Source: CAD feature listing. Evaluate the final solid. Frame: model axes, mm. A direction names the side the tool comes from. Round coordinates to 2 decimals unless told otherwise and drop trailing zeros. Order: outer loops, then holes, each group sorted by start corner. A loop starts at its lowest first (then second) coordinate and runs counter-clockwise, first axis right, second up. Notation, with made-up numbers: (19.5, -13.5) - (71.5, -13.5) arc R32 ccw to (71.5, 16.5) - close; hole circle Ø6 at (42.25, 67.25). An arc over 180 degrees is marked (long way). Put each result on its own line as item: value. Start each with the question number.
1) Access query for faces 5 (the face through (0, 0, -4)), 6 (the face through (-20, -46, 1)). Directions: +Z, -Z, +X, -X, +Y, -Y. A direction counts if a zero-diameter tool reaches every point of the face in a straight line with its end or side. Return the directions, or none.
2) Section B-B on z = -2. Output: boundary loops of the cut face in (x, y).
3) Mould query, pull axis Y, two halves, no side actions, for faces 1 (the face through (0, -72, -14)), 2 (the face through (0, 20, 3)), 3 (the face through (0, -75, -3)), 4 (the face through (1.08, -4.88, -1.97)). Classes: +Y half, -Y half, draft (parallel to the pull), parting line (faces both ways), or undercut.
4) Section A-A on z = -7. Output: boundary loops of the cut face in (x, y), then the cut area to 3 significant figures.
5) Line query: probe 1 along X at (y, z) = (-71.4, -7); probe 2 along Z at (x, y) = (10, -72.2); probe 3 along Z at (x, y) = (-10, -2). Output: solid intervals per line, ascending. Write a range as [from, to].
6) Section C-C on x = -10. Output: boundary loops of the cut face in (y, z).
7) Contact query for flat-ended pins moving along their axis: P1, Ø2.5, axis at x = 10, z = -7, coming from the -Y side; P2, Ø4, axis at x = -10, z = -7, coming from the +Y side; P3, Ø11, axis at x = -0.5, y = 0, coming from the -Z side; P4, Ø20, axis at x = -5, y = -34.5, coming from the -Z side. Output: stop coordinate, or through.
8) Section D-D on x = 0. Output: boundary loops of the cut face in (y, z), then the cut area to 3 significant figures.
```python
from build123d import *

# Parameters (mm, degrees)
BOSS_EXTRUDE1_DEPTH = 7
SKETCH2_R           = 5
BOSS_EXTRUDE2_DEPTH = 4
SKETCH3_W           = 40
SKETCH3_H           = 5
BOSS_EXTRUDE3_DEPTH = 14
SKETCH5_R           = 1.5
CUT_EXTRUDE1_DEPTH  = 6


with BuildPart() as part:
    # Sketch1 → Boss-Extrude1 (new body)
    with BuildSketch(Plane.XY):
        with BuildLine():
            Line((20, 0), (20, -75))
            Line((20, -75), (-20, -75))
            Line((-20, -75), (-20, 0))
            ThreePointArc((-20, 0), (0, 20), (20, 0))
        make_face()
    extrude(amount=BOSS_EXTRUDE1_DEPTH)

    # Sketch2 → Boss-Extrude2 (add)
    with BuildSketch(Plane(origin=(0, 0, 0), x_dir=(-1, 0, 0), z_dir=(0, 0, -1))):
        Circle(SKETCH2_R)
    extrude(amount=BOSS_EXTRUDE2_DEPTH)

    # Sketch3 → Boss-Extrude3 (add)
    with BuildSketch(Plane(origin=(0, 0, 0), x_dir=(-1, 0, 0), z_dir=(0, 0, -1))):
        with Locations((0, -72.5)):
            Rectangle(SKETCH3_W, SKETCH3_H)
    extrude(amount=BOSS_EXTRUDE3_DEPTH)

    # Sketch5 → Cut-Extrude1 (cut, through all)
    with BuildSketch(Plane(origin=(0, -70, 0), x_dir=(1, 0, 0), z_dir=(0, 1, 0))):
        with Locations((10, 7)):
            Circle(SKETCH5_R)
        with Locations((-10, 7)):
            Circle(SKETCH5_R)
    extrude(amount=-CUT_EXTRUDE1_DEPTH, mode=Mode.SUBTRACT)


solid = part.part
```
Answer sheet:
1. face 5: -Z, +X, -X, +Y
1. face 6: +Z, -Z, -X, +Y, -Y
2. outline: (-20, -75) - (20, -75) - (20, -70) - (-20, -70) - close; circle Ø10 at (0, 0)
3. face 1: draft
3. face 2: +Y half
3. face 3: -Y half
3. face 4: undercut
4. outline: (-20, -75) - (-11.5, -75) - (-11.5, -70) - (-20, -70) - close; (-8.5, -75) - (8.5, -75) - (8.5, -70) - (-8.5, -70) - close; (11.5, -75) - (20, -75) - (20, -70) - (11.5, -70) - close
4. area: 170 mm^2
5. probe 1: [-20, -11.5], [-8.5, 8.5], [11.5, 20]
5. probe 2: [-14, -8.5], [-5.5, 7]
5. probe 3: [0, 7]
6. outline: (-75, -14) - (-70, -14) - (-70, -8.5) - (-75, -8.5) - close; (-75, -5.5) - (-70, -5.5) - (-70, 0) - (17.32, 0) - (17.32, 7) - (-75, 7) - close
7. P1: through
7. P2: y = -70
7. P3: z = -4
7. P4: z = 0
8. outline: (-75, -14) - (-70, -14) - (-70, 0) - (-5, 0) - (-5, -4) - (5, -4) - (5, 0) - (20, 0) - (20, 7) - (-75, 7) - close
8. area: 775 mm^2
